from build123d import *

# Parameters (mm, degrees)
BOSS_EXTRUDE1_DEPTH     = 1
CUT_EXTRUDE3_DEPTH      = 104.456512603
CUT_EXTRUDE3_DEPTH_BACK = 104.456512603
SKETCH6_R               = 2
SKETCH2_W               = 88.5
SKETCH2_H               = 21.5
BOSS_EXTRUDE2_DEPTH     = 1
SKETCH3_W               = 1.2
SKETCH3_H               = 5.5
BOSS_EXTRUDE3_DEPTH     = 2.5
SKETCH7_W               = 8
SKETCH7_H               = 9.5
BOSS_EXTRUDE4_DEPTH     = 1
SKETCH8_R               = 1.5
CUT_EXTRUDE4_DEPTH      = 3
SKETCH9_W               = 5.5
SKETCH9_H               = 1.039758998
BOSS_EXTRUDE5_DEPTH     = 1.2
FILLET3_START           = -16
FILLET3_DEPTH           = 5.5
FILLET3_START_2         = -26.5
FILLET3_2_DEPTH         = 26.5


with BuildPart() as part:
    # Sketch1 → Boss-Extrude1 (new body)
    with BuildSketch(Plane(origin=(0, 0, 0), x_dir=(1, 0, 0), z_dir=(0, 1, 0))):
        Polygon((94.5, 18), (100, 18), (100, 8.5), (94.5, 8.5), (94.5, 0), (0, 0), (0, 26.5), (94.5, 26.5), align=None)
    extrude(amount=BOSS_EXTRUDE1_DEPTH)

    # Sketch6 → Cut-Extrude3 (cut, two sides: drawn at the far end of the back side and taken through both)
    with BuildSketch(Plane(origin=(0, 1, 0), x_dir=(1, 0, 0), z_dir=(0, 1, 0)).offset(-CUT_EXTRUDE3_DEPTH_BACK)):
        with Locations(Location((96, 13, 0), (0, 0, 270))):
            Circle(SKETCH6_R)
    extrude(amount=CUT_EXTRUDE3_DEPTH + CUT_EXTRUDE3_DEPTH_BACK, mode=Mode.SUBTRACT)

    # Sketch2 → Boss-Extrude2 (add)
    with BuildSketch(Plane(origin=(0, 1, 0), x_dir=(1, 0, 0), z_dir=(0, 1, 0))):
        with Locations((47.75, 13.25)):
            Rectangle(SKETCH2_W, SKETCH2_H)
    extrude(amount=BOSS_EXTRUDE2_DEPTH)

    # Sketch3 → Boss-Extrude3 (add)
    with BuildSketch(Plane(origin=(0, 1, 0), x_dir=(1, 0, 0), z_dir=(0, 1, 0))):
        with Locations((0.6, 13.25)):
            Rectangle(SKETCH3_W, SKETCH3_H)
    extrude(amount=BOSS_EXTRUDE3_DEPTH)

    # Sketch7 → Boss-Extrude4 (add)
    with BuildSketch(Plane(origin=(0, 1, 0), x_dir=(1, 0, 0), z_dir=(0, 1, 0))):
        with Locations((96, 13.25)):
            Rectangle(SKETCH7_W, SKETCH7_H)
    extrude(amount=BOSS_EXTRUDE4_DEPTH)

    # Sketch8 → Cut-Extrude4 (cut)
    with BuildSketch(Plane.XZ.offset(-1)):
        with Locations(Location((96, -13, 0), (0, 0, 270))):
            Circle(SKETCH8_R)
    extrude(amount=-CUT_EXTRUDE4_DEPTH, mode=Mode.SUBTRACT)

    # Sketch9 → Boss-Extrude5 (add)
    with BuildSketch(Plane.ZY):
        with Locations((-13.25, 2.980120501)):
            Rectangle(SKETCH9_W, SKETCH9_H)
    extrude(amount=BOSS_EXTRUDE5_DEPTH)

    # Fillet3: read off the stored shape, not the designer's step
    # Fillet3 outline → Fillet3 (add)
    with BuildSketch(Plane.XY.offset(FILLET3_START)):
        with BuildLine():
            Line((0, 0.627210724), (0, 2.460241002))
            Line((0, 2.460241002), (-1.2, 2.460241002))
            ThreePointArc((-1.2, 2.460241002), (-0.326679947, 1.722655839), (0, 0.627210724))
        make_face()
    extrude(amount=FILLET3_DEPTH)

    # Fillet3 2 outline → Fillet3 2 (add)
    with BuildSketch(Plane.XY.offset(FILLET3_START_2)):
        with BuildLine():
            ThreePointArc((-0.035050088, 1), (-0.008781802, 0.814427412), (0, 0.627210724))
            Line((0, 0.627210724), (0, 1))
            Line((0, 1), (-0.035050088, 1))
        make_face()
    extrude(amount=FILLET3_2_DEPTH)


solid = part.part
Read the model definition and answer for the solid it produces. Units are mm, in the model's axes. A direction names the side the tool comes from. Coordinates: 2 decimals unless noted, no trailing zeros. Write each loop counter-clockwise with the first axis right and the second up, starting at its lowest first coordinate (ties: lowest second). Pieces come first, ordered by that corner, then holes. Notation, with made-up numbers: (71, 68.5) -> (112, 68.5) arc R21 cw to (112, 76.5) -> close; hole circle Ø1 at (-8.75, -38). An arc over 180 degrees is marked (long way). Return JSON: item names as keys, results as strings.
(1) The part is cut by section D-D on z = -6. Give the vertices of the cut face in (x, y), then the cut area to 3 significant figures.
Answers below:
{"outline": "(-0.04, 1) arc R2 cw to (0, 0.63) -> (0, 0) -> (94.5, 0) -> (94.5, 1) -> (92, 1) -> (92, 2) -> (3.5, 2) -> (3.5, 1) -> close", "area": "183 mm^2"}
(2) The part is cut by section A-A on z = -13. Give the vertices of the cut face in (x, y).
Answers below:
{"outline": "(-1.2, 2.46) arc R2 cw to (0, 0.63) -> (0, 0) -> (94, 0) -> (94, 1) -> (94.5, 1) -> (94.5, 2) -> (3.5, 2) -> (3.5, 1) -> (1.2, 1) -> (1.2, 3.5) -> (-1.2, 3.5) -> close; (97.5, 1) -> (98, 1) -> (98, 0) -> (100, 0) -> (100, 2) -> (97.5, 2) -> close"}
(3) Consider line 1 along X through (y, z) = (0.65, -13); line 2 along Z through (x, y) = (96, 1.55); line 3 along X through (y, z) = (1.85, -13). Determine where each line is inside the solid, lowest interval first. Write a range as from..to.
Answers below:
{"line 1": "0..94, 98..100", "line 2": "-18..-14.5, -11.5..-8.5", "line 3": "-0.42..1.2, 3.5..94.5, 97.5..100"}
(4) For a pull along X with two mould halves and no side action, classify faces 4 (the cylindrical face through (97.487, 1.493, -12.805)), 5 (the flat face through (100, 1, -13)), 6 (the flat face through (0, 3.5, -13)) as pulls with the +X half, pulls with the -X half, needs draft (parallel to the pull), parting line crosses it, or undercut.
Answers below:
{"face 4": "undercut", "face 5": "pulls with the +X half", "face 6": "needs draft"}
(5) Each of these flat-tipped pins is pushed along its axis until it touches: P1, Ø0.5, axis at y = 0.5, z = -6, coming from the +X side; P2, Ø13, axis at x = 47.5, z = -7.5, coming from the +Y side; P3, Ø1.8, axis at x = 96, z = -13, coming from the +Y side; P4, Ø0.5, axis at x = 33, y = 1.5, coming from the -Z side. Where does it stop, or does it pass through?
Answers below:
{"P1": "x = 94.5", "P2": "y = 2", "P3": "through", "P4": "z = -24"}
(6) The part is cut by section C-C on x = 52. Give the vertices of the cut face in (y, z).
Answers below:
{"outline": "(0, -26.5) -> (1, -26.5) -> (1, -24) -> (2, -24) -> (2, -2.5) -> (1, -2.5) -> (1, 0) -> (0, 0) -> close"}
(7) Which of the six approach directions +Z, -Z, +X, -X, +Y, -Y give full straight-line access (tool end or side, diameter ignored) to faces 1 (the flat face through (0, 3, -16)), 2 (the flat face through (51, 2, -13)), 3 (the flat face through (0, 3, -10.5))?
Answers below:
{"face 1": "-Z, -X, +Y", "face 2": "+Z, -Z, +X, +Y", "face 3": "+Z, -X, +Y"}
(8) The part is cut by section B-B on x = 96. Give the vertices of the cut face in (y, z).
Answers below:
{"outline": "(0, -18) -> (2, -18) -> (2, -14.5) -> (1, -14.5) -> (1, -15) -> (0, -15) -> close; (0, -11) -> (1, -11) -> (1, -11.5) -> (2, -11.5) -> (2, -8.5) -> (0, -8.5) -> close"}
